Verification items for this drawing (mm, ordinates from the low corner). A direction names the side the tool comes from. Round coordinates to 2 decimals unless told otherwise and drop trailing zeros.
Item 1: Scan lines: probe 1 along X at (y, z) = (93.5, 10.5); probe 2 along Z at (x, y) = (79, 78.5); probe 3 along X at (y, z) = (44.5, 20). Record each from-to range of solid material in increasing order.
Item 2: Access from +Z, -Z, +X, -X, +Y, -Y to the whole of each face (thin tool, end or side, straight path). Record for the marked faces 1 and 2.
Item 3: Depth check by flat-ended pin: P1, Ø5, axis at x = 137, z = 38, coming from the -Y side (1 decimal); P2, Ø5, axis at x = 130, z = 32.5, coming from the -Y side; P3, Ø4, axis at x = 109, z = 34, coming from the +Y side. Enter the tip coordinate at first touch or a pass-through.
Item 4: Draft check along Y on the marked faces 3, 4 and 5. Enter one of: pulls with the +Y half, pulls with the -Y half, needs draft (parallel to the pull), parting line crosses it, or undercut.
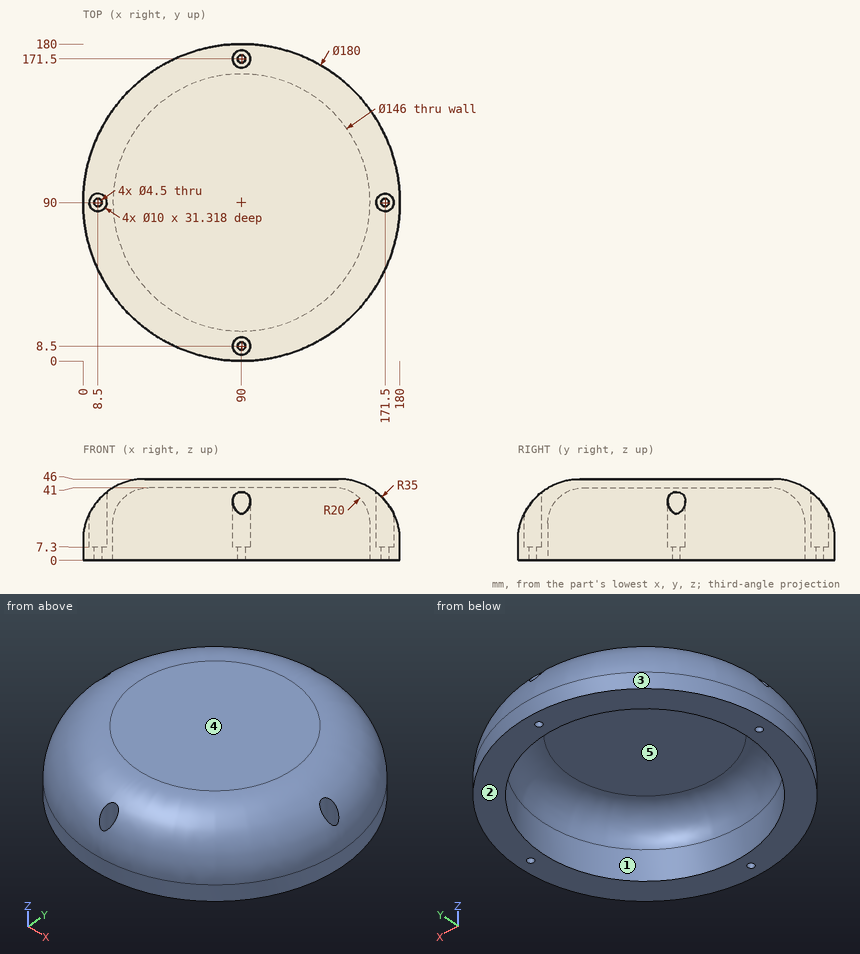
Resolved:
1. probe 1: x = 0.07 to 4.93, 12.07 to 17.08, 162.92 to 167.93, 175.07 to 179.93
1. probe 2: z = 41 to 46
1. probe 3: x = 13.72 to 32.91, 147.09 to 166.28
2. face 1: -Z
2. face 2: -Z, +X, -X, +Y, -Y
3. P1: stops at y = 24.8
3. P2: stops at y = 15.27
3. P3: stops at y = 170.86
4. face 3: parting line crosses it
4. face 4: needs draft
4. face 5: undercut
